Can you work these out from the model? Positions are in its coordinate system, mm. A direction names the side the tool comes from. Coordinates: 2 decimals unless noted, no trailing zeros. Loops run counter-clockwise (first coordinate to the right, second up) from the corner with the lowest first, then second, coordinate; pieces in that order, holes last. Notation, with made-up numbers: (34.25, 78.5) - (45.25, 78.5) arc R30 cw to (45.25, 108.5) - close; hole circle Ø4 at (5.25, 24.25). An arc over 180 degrees is marked (long way). Put each result on its own line as item: value. Start each with the question number.
from build123d import *

# Parameters (mm, degrees)
SKETCH1_R           = 27
BOSS_EXTRUDE1_DEPTH = 5
SKETCH2_R           = 27
SKETCH2_R_2         = 25
BOSS_EXTRUDE2_DEPTH = 160
SKETCH3_R           = 5
CUT_EXTRUDE1_DEPTH  = 160
SKETCH4_R           = 10
CUT_EXTRUDE6_DEPTH  = 41


with BuildPart() as part:
    # Sketch1 → Boss-Extrude1 (new body)
    with BuildSketch(Plane(origin=(0, 0, 0), x_dir=(1, 0, 0), z_dir=(0, 1, 0))):
        Circle(SKETCH1_R)
    extrude(amount=BOSS_EXTRUDE1_DEPTH)

    # Sketch2 → Boss-Extrude2 (add)
    with BuildSketch(Plane(origin=(0, 5, 0), x_dir=(1, 0, 0), z_dir=(0, 1, 0))):
        Circle(SKETCH2_R)
        Circle(SKETCH2_R_2, mode=Mode.SUBTRACT)
    extrude(amount=BOSS_EXTRUDE2_DEPTH)

    # Sketch3 → Cut-Extrude1 (cut)
    with BuildSketch(Plane.XY):
        with Locations((0, 20)):
            Circle(SKETCH3_R)
    extrude(amount=-CUT_EXTRUDE1_DEPTH, mode=Mode.SUBTRACT)

    # Sketch4 → Cut-Extrude6 (cut)
    with BuildSketch(Plane.XY):
        with Locations((0, 65)):
            Circle(SKETCH4_R)
    extrude(amount=CUT_EXTRUDE6_DEPTH, mode=Mode.SUBTRACT)


solid = part.part
Q1. I want a section at C-C on y = 34. List the corners of the cut face in (x, z) for me, and give its area (3 significant figures).
Q2. Please list where these lines run through material, in increasing order: line 1 along X through (y, z) = (57, 0); line 2 along Y through (x, z) = (0, -26); line 3 along Y through (x, z) = (0, 24.95). Write a range as [from, to].
Q3. I want a section at D-D on x = -7. List the corners of the cut face in (y, z) for me.
Q4. I want a section at B-B on x = 0. List the corners of the cut face in (y, z) for me.
Q5. I want a section at A-A on z = 0. List the corners of the cut face in (x, y) for me, and give its area (3 significant figures).
Q6. We'd pull the mould along Z, two halves only. Please class faces 5 (the flat face through (0, 0, 0)), 6 (the cylindrical face through (13.44, 83.88, -21.08)), 7 (the cylindrical face through (-3.51, 81.34, -26.77)): released by +Z, released by -Z, zero draft, split by the parting line, or undercut.
Q7. Will these pins go through, and if not, where does the flat tip stop? pin 1 (1 mm diameter, centred on y = 51.5, z = 6, fed in from +X); pin 2 (4 mm diameter, centred on x = -13.5, z = 12.5, fed in from +Y); pin 3 (3 mm diameter, centred on x = 19.5, y = 96, fed in from -Z).
Q8. On a 3-axis mill with a long thin cutter (end or side, diameter ignored), from which of +Z, -Z, +X, -X, +Y, -Y can I reach the whole of each face in a straight line? I mean faces 1 (the flat face through (0, 5, 0)), 2 (the cylindrical face through (4.619, 18.085, -25.73)), 3 (the flat face through (24, 165, 8)), 4 (the cylindrical face through (-7.37, 71.76, 24.93)). Say none if no direction works.
Calculated:
1. outline: circle Ø54 at (0, 0); hole circle Ø50 at (0, 0)
1. area: 327 mm2
2. line 1: [-27, -25], [25, 27]
2. line 2: [0, 15], [25, 165]
2. line 3: [0, 5]
3. outline: (0, -26.08) - (165, -26.08) - (165, -24) - (5, -24) - (5, 24) - (57.86, 24) - (57.86, 26.08) - (0, 26.08) - close; (72.14, 24) - (165, 24) - (165, 26.08) - (72.14, 26.08) - close
4. outline: (0, -27) - (15, -27) - (15, -25) - (5, -25) - (5, 25) - (55, 25) - (55, 27) - (0, 27) - close; (25, -27) - (165, -27) - (165, -25) - (25, -25) - close; (75, 25) - (165, 25) - (165, 27) - (75, 27) - close
5. outline: (-27, 0) - (27, 0) - (27, 165) - (25, 165) - (25, 5) - (-25, 5) - (-25, 165) - (-27, 165) - close
5. area: 910 mm2
6. face 5: zero draft
6. face 6: undercut
6. face 7: split by the parting line
7. pin 1: x = 26.43
7. pin 2: y = 5
7. pin 3: z = -20.12
8. face 1: +Y
8. face 2: -Z
8. face 3: +Z, -Z, +X, -X, +Y
8. face 4: +Z
